from build123d import *

# Parameters (mm, degrees)
SKETCH1_W            = 12.8
SKETCH1_H            = 9.5
BOSS_EXTRUDE1_DEPTH  = 3.5
SKETCH2_R            = 3
BOSS_EXTRUDE2_DEPTH  = 8
SKETCH4_R            = 1.3
BOSS_EXTRUDE3_DEPTH  = 10
FILLET1_R            = 1
FILLET1_OF_MIRROR1_R = 1
SKETCH5_R            = 0.6
BOSS_EXTRUDE4_DEPTH  = 6


with BuildPart() as part:
    # Sketch1 → Boss-Extrude1 (new, symmetric)
    with BuildSketch(Plane(origin=(0, 0, 0), x_dir=(1, 0, 0), z_dir=(0, 1, 0))):
        Rectangle(SKETCH1_W, SKETCH1_H)
    extrude(amount=BOSS_EXTRUDE1_DEPTH, both=True)

    # Sketch2 → Boss-Extrude2 (add)
    with BuildSketch(Plane.XY.offset(4.75)):
        with Locations(Location((0, 0, 0), (0, 0, 180))):
            Circle(SKETCH2_R)
    extrude(amount=BOSS_EXTRUDE2_DEPTH)

    # Sketch4 → Boss-Extrude3 (add)
    with BuildSketch(Plane(origin=(3.457717226, 0, 19.75), x_dir=(0.9396926207859079, 0, -0.34202014332567043), z_dir=(0.34202014332567043, 0, 0.9396926207859079))):
        Circle(SKETCH4_R)
    boss_extrude3 = extrude(amount=-BOSS_EXTRUDE3_DEPTH)

    # Fillet1
    fillet1_edges = [part.edges().sort_by_distance(p)[0] for p in [
        (2.236116819, 0, 20.194626186),
    ]]
    fillet(fillet1_edges, radius=FILLET1_R)

    # Mirror1: Boss-Extrude3 across plane
    add(boss_extrude3.mirror(Plane(origin=(0, 0, 0), x_dir=(0, 0, 1), z_dir=(1, 0, 0))))

    # Fillet1 of Mirror1
    fillet1_of_mirror1_edges = [part.edges().sort_by_distance(p)[0] for p in [
        (-2.236116819, 0, 20.194626186),
    ]]
    fillet(fillet1_of_mirror1_edges, radius=FILLET1_OF_MIRROR1_R)

    # Sketch5 → Boss-Extrude4 (add)
    with BuildSketch(Plane(origin=(0, 0, -4.75), x_dir=(-1, 0, 0), z_dir=(0, 0, -1))):
        with Locations(Location((0, 0, 0), (0, 0, 180))):
            Circle(SKETCH5_R)
        with Locations(Location((-4.5, 0, 0), (0, 0, 180))):
            Circle(SKETCH5_R)
        with Locations(Location((4.5, 0, 0), (0, 0, 180))):
            Circle(SKETCH5_R)
    extrude(amount=BOSS_EXTRUDE4_DEPTH)


solid = part.part
Geometry: final body of the model. Coordinates: model frame, mm. A direction names the side the tool comes from. Round coordinates to 2 decimals unless told otherwise and drop trailing zeros. Order: outer loops, then holes, each group sorted by start corner. A loop starts at its lowest first (then second) coordinate and runs counter-clockwise, first axis right, second up.
Q1. Access query for faces 1 (the face through (0.323, -0.506, -7.708)), 2 (the face through (0, 3.5, 0)), 3 (the face through (-2.86, -0.9, 8.69)). Directions: +Z, -Z, +X, -X, +Y, -Y. A direction counts if a zero-diameter tool reaches every point of the face in a straight line with its end or side. Return the directions, or none.
Result sheet:
face 1: -Z
face 2: +Z, -Z, +X, -X, +Y
face 3: none
Q2. Section C-C, the plane z = 6.5. Output: boundary loops of the cut face in (x, y).
Result sheet:
outline: circle Ø6 at (0, 0)
Q3. Pin query (flat end, axial travel): pin 1 (2 mm diameter, centred on x = 3, y = -1, fed in from -Z); pin 2 (6 mm diameter, centred on x = 3.5, z = 11.5, fed in from +Y); pin 3 (2 mm diameter, centred on y = 1, z = 9.5, fed in from -X). Return the tip coordinate at first contact, or that it passes through.
Result sheet:
pin 1: stops at z = -4.75
pin 2: stops at y = 2.96
pin 3: stops at x = -3
Q4. Mould query, pull axis Z, two halves, no side actions, for faces 4 (the face through (0, 1.3, 12.75)), 5 (the face through (4.5, 0, -10.75)), 6 (the face through (3.9, 0, -7.7)). Classes: released by +Z, released by -Z, zero draft, split by the parting line, or undercut.
Result sheet:
face 4: undercut
face 5: released by -Z
face 6: zero draft
Q5. Material intervals for probe 1 along Z at (x, y) = (-2.5, -1.5); probe 2 along Z at (x, y) = (3.25, 2); probe 3 along X at (y, z) = (1, 6.5), sorted ascending.
Result sheet:
probe 1: z = -4.75 to 12.75
probe 2: z = -4.75 to 4.75
probe 3: x = -2.83 to 2.83
Q6. Section B-B, the plane y = 2.5. Output: boundary loops of the cut face in (x, z), and give its area (3 significant figures).
Result sheet:
outline: (-6.4, -4.75) - (6.4, -4.75) - (6.4, 4.75) - (1.66, 4.75) - (1.66, 12.75) - (-1.66, 12.75) - (-1.66, 4.75) - (-6.4, 4.75) - close
area: 148 mm2
Q7. Section A-A, the plane z = -6. Output: boundary loops of the cut face in (x, y).
Result sheet:
outline: circle Ø1.2 at (-4.5, 0); circle Ø1.2 at (0, 0); circle Ø1.2 at (4.5, 0)
